```python
from build123d import *

# Parameters (mm, degrees)
SKETCH1_W           = 19.05
SKETCH1_H           = 19.05
BOSS_EXTRUDE1_DEPTH = 6.35
SKETCH2_R           = 2
CUT_EXTRUDE1_DEPTH  = 28.679008291
CUT_EXTRUDE2_DEPTH  = 28.679008291


with BuildPart() as part:
    # Sketch1 → Boss-Extrude1 (new body)
    with BuildSketch(Plane.XY):
        with Locations((9.525, 9.525)):
            Rectangle(SKETCH1_W, SKETCH1_H)
    extrude(amount=BOSS_EXTRUDE1_DEPTH)

    # Sketch2 → Cut-Extrude1 (cut, through all)
    with BuildSketch(Plane.XZ):
        with Locations(Location((2.54, 3.175, 0), (0, 0, 270))):
            Circle(SKETCH2_R)
        with Locations(Location((16.51, 3.175, 0), (0, 0, 270))):
            Circle(SKETCH2_R)
    extrude(amount=-CUT_EXTRUDE1_DEPTH, mode=Mode.SUBTRACT)

    # Sketch3 → Cut-Extrude2 (cut, through all)
    with BuildSketch(Plane.XY.offset(6.35)):
        with BuildLine():
            ThreePointArc((11.811, 13.97), (9.525, 16.256), (7.239, 13.97))
            Line((7.239, 13.97), (11.811, 13.97))
        make_face()
        with BuildLine():
            Line((11.811, 13.97), (7.239, 13.97))
            ThreePointArc((7.239, 13.97), (9.525, 11.684), (11.811, 13.97))
        make_face()
        with BuildLine():
            ThreePointArc((11.811, 13.97), (9.525, 11.684), (7.239, 13.97))
            Line((7.239, 13.97), (7.239, 5.08))
            ThreePointArc((7.239, 5.08), (9.525, 7.366), (11.811, 5.08))
            Line((11.811, 5.08), (11.811, 13.97))
        make_face()
        with BuildLine():
            ThreePointArc((11.811, 5.08), (9.525, 7.366), (7.239, 5.08))
            Line((7.239, 5.08), (11.811, 5.08))
        make_face()
        with BuildLine():
            Line((11.811, 5.08), (7.239, 5.08))
            ThreePointArc((7.239, 5.08), (9.525, 2.794), (11.811, 5.08))
        make_face()
    extrude(amount=-CUT_EXTRUDE2_DEPTH, mode=Mode.SUBTRACT)


solid = part.part
```
Here's how the part is built. I have some questions about the finished solid (model axes, mm). A direction names the side the tool comes from. Coordinates: 2 decimals unless noted, no trailing zeros. Order: outer loops, then holes, each group sorted by start corner. A loop starts at its lowest first (then second) coordinate and runs counter-clockwise, first axis right, second up. Notation, with made-up numbers: (12, 6.25) - (32, 6.25) arc R17 cw to (32, 10.25) - close; hole circle Ø4 at (-14.75, 62). An arc over 180 degrees is marked (long way). One line per question, with ' | ' between items. Start each with the question number.
1. If we section it at D-D (z = 3): Write out the boundary of the cut face in (x, y) (3 decimals).
2. If we mould it in two halves opening along Y, with no side actions, what happens to faces 3 (the flat face through (11.811, 9, 3)), 4 (the flat face through (9, 19.05, 3)), 5 (the flat face through (14, 10, 0)), 6 (the cylindrical face through (9.575, 16.255, 3.219))? For each: released by +Y, released by -Y, zero draft, split by the parting line, or undercut.
3. I'm going to push a flat-ended pin straight in: pin 1 Ø2.5 at (x, z) = (2.54, 3.175) entering from +Y. Where does the tip first touch, or does it pass through?
4. If we section it at C-C (z = 5.75): Write out the boundary of the cut face in (x, y) (3 decimals), and give its area (3 significant figures).
5. Please list where these lines run through material, in increasing order: line 1 along X through (y, z) = (9, 5.5); line 2 along X through (y, z) = (4.5, 1.5); line 3 along X through (y, z) = (12, 4.75). Write a range as [from, to].
6. If we section it at B-B (x = 16.51): Write out the boundary of the cut face in (y, z) (3 decimals).
7. Which directions (+Z, -Z, +X, -X, +Y, -Y) give clear straight access to the entire face, cutting with the end or side of a thin tool? Please do faces 1 (the flat face through (9, 0, 3)), 2 (the flat face through (7.239, 10, 3)).
8. If we section it at A-A (y = 11.25): Write out the boundary of the cut face in (x, z) (3 decimals).
Model answer:
1) outline: (0, 0) - (0.548, 0) - (0.548, 19.05) - (0, 19.05) - close; (4.532, 0) - (14.518, 0) - (14.518, 19.05) - (4.532, 19.05) - close; (18.502, 0) - (19.05, 0) - (19.05, 19.05) - (18.502, 19.05) - close; hole (7.239, 5.08) arc R2.286 ccw to (11.811, 5.08) - (11.811, 13.97) arc R2.286 ccw to (7.239, 13.97) - close
2) face 3: undercut | face 4: released by +Y | face 5: zero draft | face 6: undercut
3) pin 1: passes through
4) outline: (0, 0) - (19.05, 0) - (19.05, 19.05) - (0, 19.05) - close; hole (7.239, 5.08) arc R2.286 ccw to (11.811, 5.08) - (11.811, 13.97) arc R2.286 ccw to (7.239, 13.97) - close | area: 306 mm²
5) line 1: x = [0, 7.24], [11.81, 19.05] | line 2: x = [0, 1.45], [3.63, 7.31], [11.74, 15.42], [17.6, 19.05] | line 3: x = [0, 1.31], [3.77, 7.24], [11.81, 15.28], [17.74, 19.05]
6) outline: (0, 0) - (19.05, 0) - (19.05, 1.175) - (0, 1.175) - close; (0, 5.175) - (19.05, 5.175) - (19.05, 6.35) - (0, 6.35) - close
7) face 1: +Z, -Z, +X, -X, -Y | face 2: +Z, -Z
8) outline: (0, 0) - (7.239, 0) - (7.239, 6.35) - (0, 6.35) - close; (11.811, 0) - (19.05, 0) - (19.05, 6.35) - (11.811, 6.35) - close; hole circle Ø4 at (2.54, 3.175); hole circle Ø4 at (16.51, 3.175)
